```python
from build123d import *

# Parameters (mm, degrees)
SKETCH1_R           = 2.2
BOSS_EXTRUDE1_DEPTH = 2.38125
SKETCH2_W           = 3.175
SKETCH2_H           = 26.985
BOSS_EXTRUDE2_DEPTH = 28.575
SKETCH3_W           = 26.985
SKETCH3_H           = 3.175
BOSS_EXTRUDE3_DEPTH = 9.525
SKETCH4_W           = 26.985
SKETCH4_H           = 3.175
BOSS_EXTRUDE4_DEPTH = 9.525
FILLET1_R           = 3.175
SKETCH5_R           = 2.159
CUT_EXTRUDE1_DEPTH  = 3.175


with BuildPart() as part:
    # Sketch1 → Boss-Extrude1 (new body)
    with BuildSketch(Plane(origin=(0, 0, 0), x_dir=(1, 0, 0), z_dir=(0, 1, 0))):
        Polygon((20.15, 0), (-20.15, 0), (-20.15, 20), (-31.52, 20), (-31.52, -6.985), (31.52, -6.985), (31.52, 20), (20.15, 20), align=None)
        with Locations(Location((-23.9, 15.1, 0), (0, 0, 90))):
            Circle(SKETCH1_R, mode=Mode.SUBTRACT)
        with Locations(Location((-23.9, 4.9, 0), (0, 0, 90))):
            Circle(SKETCH1_R, mode=Mode.SUBTRACT)
        with Locations(Location((23.9, 4.9, 0), (0, 0, 90))):
            Circle(SKETCH1_R, mode=Mode.SUBTRACT)
        with Locations(Location((23.9, 15.1, 0), (0, 0, 90))):
            Circle(SKETCH1_R, mode=Mode.SUBTRACT)
    extrude(amount=BOSS_EXTRUDE1_DEPTH)

    # Sketch2 → Boss-Extrude2 (add)
    with BuildSketch(Plane.XZ):
        with Locations((29.9325, -6.5075)):
            Rectangle(SKETCH2_W, SKETCH2_H)
        with Locations((-29.9325, -6.5075)):
            Rectangle(SKETCH2_W, SKETCH2_H)
    extrude(amount=BOSS_EXTRUDE2_DEPTH)

    # Sketch3 → Boss-Extrude3 (add)
    with BuildSketch(Plane(origin=(31.52, 0, 0), x_dir=(0, 0, -1), z_dir=(1, 0, 0))):
        with Locations((6.5075, -26.9875)):
            Rectangle(SKETCH3_W, SKETCH3_H)
    extrude(amount=BOSS_EXTRUDE3_DEPTH)

    # Sketch4 → Boss-Extrude4 (add)
    with BuildSketch(Plane.ZY.offset(31.52)):
        with Locations((-6.5075, -26.9875)):
            Rectangle(SKETCH4_W, SKETCH4_H)
    extrude(amount=BOSS_EXTRUDE4_DEPTH)

    # Fillet1
    fillet1_edges = [part.edges().sort_by_distance(p)[0] for p in [
        (41.045, -26.9875, 6.985),
        (41.045, -26.9875, -20),
        (-41.045, -26.9875, -20),
        (-41.045, -26.9875, 6.985),
    ]]
    fillet(fillet1_edges, radius=FILLET1_R)

    # Sketch5 → Cut-Extrude1 (cut)
    with BuildSketch(Plane(origin=(0, -25.4, 0), x_dir=(1, 0, 0), z_dir=(0, 1, 0))):
        with Locations(Location((36.2825, -2.2225, 0), (0, 0, 270))):
            Circle(SKETCH5_R)
        with Locations(Location((36.2825, 15.2375, 0), (0, 0, 270))):
            Circle(SKETCH5_R)
        with Locations(Location((-36.2825, -2.2225, 0), (0, 0, 270))):
            Circle(SKETCH5_R)
        with Locations(Location((-36.2825, 15.2375, 0), (0, 0, 270))):
            Circle(SKETCH5_R)
    extrude(amount=-CUT_EXTRUDE1_DEPTH, mode=Mode.SUBTRACT)


solid = part.part
```
CAD build for the part. Positions are in the model's coordinates, mm. A direction names the side the tool comes from. Coordinates: 2 decimals unless noted, no trailing zeros. Loops run counter-clockwise (first coordinate to the right, second up) from the corner with the lowest first, then second, coordinate; pieces in that order, holes last. Notation, with made-up numbers: (73.5, 23.5) - (94.5, 23.5) arc R18 ccw to (94.5, 35.5) - close; hole circle Ø4 at (-40, -32). An arc over 180 degrees is marked (long way). Return JSON: item names as keys, results as strings.
1. Band-saw the part on D-D (z = -4.9). Give the cut face in (x, y) (3 decimals), and give its area (3 significant figures).
Result:
{"outline": "(-41.045, -28.575) - (-28.345, -28.575) - (-28.345, 0) - (-26.1, 0) - (-26.1, 2.381) - (-31.52, 2.381) - (-31.52, -25.4) - (-41.045, -25.4) - close; (-21.7, 0) - (-20.15, 0) - (-20.15, 2.381) - (-21.7, 2.381) - close; (20.15, 0) - (21.7, 0) - (21.7, 2.381) - (20.15, 2.381) - close; (26.1, 0) - (28.345, 0) - (28.345, -28.575) - (41.045, -28.575) - (41.045, -25.4) - (31.52, -25.4) - (31.52, 2.381) - (26.1, 2.381) - close", "area": "275 mm2"}
2. Band-saw the part on B-B (x = -23.9). Give the cut face in (y, z) (3 decimals).
Result:
{"outline": "(0, -20) - (2.381, -20) - (2.381, -17.3) - (0, -17.3) - close; (0, -12.9) - (2.381, -12.9) - (2.381, -7.1) - (0, -7.1) - close; (0, -2.7) - (2.381, -2.7) - (2.381, 6.985) - (0, 6.985) - close"}
3. Probe L1, parallel to X at y = 1.35, z = -4.9; L2, parallel to Z at x = -23.9, y = 1.4 (3 decimals); L3, parallel to X at y = -21, z = -7.75 (3 decimals). List the from-to ranges inside material, lowest first. Write a range as from..to.
Result:
{"L1": "x = -31.52..-26.1, -21.7..-20.15, 20.15..21.7, 26.1..31.52", "L2": "z = -20..-17.3, -12.9..-7.1, -2.7..6.985", "L3": "x = -31.52..-28.345, 28.345..31.52"}
4. 3-axis set-ups, long thin cutter, end or side, ignore diameter. For faces 1 (the cylindrical face through (-34.142, -26.965, -15.519)), 2 (the flat face through (28.345, -14, -7)), 3 (the flat face through (20.15, 1, -10)), 4 (the flat face through (31.52, -11, -7)), 5 (the flat face through (-36, -25.4, -7)): which of +Z, -Z, +X, -X, +Y, -Y reach the whole face in a straight line?
Result:
{"face 1": "+Y, -Y", "face 2": "+Z, -Z, -Y", "face 3": "-Z, +Y, -Y", "face 4": "+Z, -Z, +X, +Y", "face 5": "+Z, -Z, -X, +Y"}
5. Band-saw the part on A-A (z = -8.75). Give the cut face in (x, y) (3 decimals).
Result:
{"outline": "(-41.045, -28.575) - (-28.345, -28.575) - (-28.345, 0) - (-20.15, 0) - (-20.15, 2.381) - (-31.52, 2.381) - (-31.52, -25.4) - (-41.045, -25.4) - close; (20.15, 0) - (28.345, 0) - (28.345, -28.575) - (41.045, -28.575) - (41.045, -25.4) - (31.52, -25.4) - (31.52, 2.381) - (20.15, 2.381) - close"}
6. Band-saw the part on C-C (y = -22.5). Give the cut face in (x, z) (3 decimals).
Result:
{"outline": "(-31.52, -20) - (-28.345, -20) - (-28.345, 6.985) - (-31.52, 6.985) - close; (28.345, -20) - (31.52, -20) - (31.52, 6.985) - (28.345, 6.985) - close"}
7. Mould opens along Z. For faces 6 (the flat face through (0, 2.381, 2)), 7 (the flat face through (0, 1, 0)), 8 (the cylindrical face through (38.423, -26.965, -15.519)) say: released by +Z, released by -Z, zero draft, split by the parting line, or undercut.
Result:
{"face 6": "zero draft", "face 7": "released by -Z", "face 8": "undercut"}
8. Drop flat-ended pins along their axis: pin 1 (1.5 mm diameter, centred on y = -2.5, z = -5.5, fed in from -X); pin 2 (12 mm diameter, centred on x = -12.5, z = -3.5, fed in from -Y); pin 3 (12 mm diameter, centred on x = -16.5, y = -10.5, fed in from -Z); pin 4 (8 mm diameter, centred on y = -13.5, z = -1.5, fed in from +X). Give the stop position or say it passes through.
Result:
{"pin 1": "stops at x = -31.52", "pin 2": "stops at y = 0", "pin 3": "passes through", "pin 4": "stops at x = 31.52"}
